Autodesk Inventor part; units mm, degrees
ref_plane "YZ Plane" through (0, 0, 0) normal (1, 0, 0) x (0, 1, 0)
ref_plane "XZ Plane" through (0, 0, 0) normal (0, 1, 0) x (-1, 0, 0)
ref_plane "XY Plane" through (0, 0, 0) normal (0, 0, 1) x (1, 0, 0)
sketch "Sketch1" plane through (0, 0, 0) normal (0, 1, 0) x (-1, 0, 0)
  circle A0 centre (0, 0) radius 10
  line L0 (0, 0) -> (10, 0)
  line L1 (0, 0) -> (0, -10)
  line L2 (10, 0) -> (9, 0)
  line L3 (0, -10) -> (0, -9)
  circle A1 centre (9, 0) radius 0.5
  circle A2 centre (0, -9) radius 0.5
  dimension "d0" = 20
  dimension "d1" = 1
  dimension "d2" = 1
  dimension "d3" = 1
  dimension "d4" = 1
extrude "Extrusion1" add sketch "Sketch1" along normal blind 2 contours L0 A1 L1 A2 A0 | A0 L1 A2 L0 A1
sketch "Sketch2" plane through (0, 2, 0) normal (0, 1, 0) x (1, 0, 0)
  line L0 (0, 0) -> (-7.0711, 7.0711)
  circle A0 centre (0, 0) radius 10
  line L1 (0, 0) -> (10, 0) construction
  line L2 (-7.0711, 7.0711) -> (-6.364, 6.364)
  circle A1 centre (-6.364, 6.364) radius 0.5
  dimension "d7" = 135
  dimension "d8" = 1
  dimension "d9" = 1
extrude "Extrusion2" cut sketch "Sketch2" against normal blind 10 contours A1 L0 | L0 A1
sketch "Sketch3" plane through (0, 2, 0) normal (0, 1, 0) x (1, 0, 0)
  line L0 (0, 0) -> (7.0711, 7.0711)
  line L1 (0, 0) -> (10, 0) construction
  line L2 (7.0711, 7.0711) -> (6.364, 6.364)
  circle A0 centre (6.364, 6.364) radius 0.5
  dimension "d12" = 10
  dimension "d13" = 45
  dimension "d14" = 1
  dimension "d15" = 1
extrude "Extrusion3" cut sketch "Sketch3" against normal blind 10
properties part number "drum"
Here's how the part is built. I have some questions about the finished solid (model axes, mm). Give positions to 0.01 mm unless a question says otherwise; leave off trailing zeros. Order: outer loops, then holes, each group sorted by start corner. A loop starts at its lowest first (then second) coordinate and runs counter-clockwise, first axis right, second up. Notation, with made-up numbers: M 46.5,9.25 L 72.5,9.25 A26 cw 72.5,42.25 Z; hole C -7.75,40 d11. An arc over 180 degrees is marked long. Answer as a JSON object with one key per item and string values. Group by question number.
1) We'd pull the mould along Z, two halves only. Please class faces 1 (the flat face through (0, 0, 0)), 2 (the cylindrical face through (2.17, 0.99, 9.76)), 3 (the cylindrical face through (-9.462, 0.986, 0.192)): pulls with the +Z half, pulls with the -Z half, needs draft (parallel to the pull), parting line crosses it, or undercut.
2) Please list where these lines run through material, in increasing order: L1, parallel to Z at x = 0, y = 1.35; L2, parallel to X at y = 1.95, z = -6.5; L3, parallel to Z at x = -9, y = 1.35. Write a range as [from, to].
3) Suppose I cut it at C-C, the plane y = 1.2. Write out the boundary of the cut face in (x, z), plus the area to 3 significant figures.
4) Suppose I cut it at D-D, the plane x = 5.25. Write out the boundary of the cut face in (y, z), plus the area to 3 significant figures.
5) Suppose I cut it at A-A, the plane z = 0. Write out the boundary of the cut face in (x, y), plus the area to 3 significant figures.
6) I'm going to push flat-ended pins straight in: pin 1 Ø1 at (x, y) = (1, 1) entering from +Z; pin 2 Ø1.5 at (x, z) = (-2.5, 7.5) entering from -Y. Where does each tip first touch, or does it pass through?
7) Suppose I cut it at B-B, the plane x = 0. Write out the boundary of the cut face in (y, z), plus the area to 3 significant figures.
Results found:
{
 "1": {"face 1": "needs draft", "face 2": "parting line crosses it", "face 3": "undercut"},
 "2": {"L1": "[-10, -9.5], [-8.5, 10]", "L2": "[-7.6, -6.85], [-5.88, 5.88], [6.85, 7.6]", "L3": "[-4.36, -0.5], [0.5, 4.36]"},
 "3": {"outline": "C 0,0 d20; hole C -9,0 d1; hole C -6.36,-6.36 d1; hole C 0,-9 d1; hole C 6.36,-6.36 d1", "area": "311 mm²"},
 "4": {"outline": "M 0,-8.51 L 2,-8.51 L 2,8.51 L 0,8.51 Z", "area": "34.0 mm²"},
 "5": {"outline": "M -10,0 L -9.5,0 L -9.5,2 L -10,2 Z; M -8.5,0 L 10,0 L 10,2 L -8.5,2 Z", "area": "38.0 mm²"},
 "6": {"pin 1": "z = 9.99", "pin 2": "y = 0"},
 "7": {"outline": "M 0,-10 L 2,-10 L 2,-9.5 L 0,-9.5 Z; M 0,-8.5 L 2,-8.5 L 2,10 L 0,10 Z", "area": "38.0 mm²"}
}
